Verification items for the finished model (mm, model axes). A direction names the side the tool comes from. Round coordinates to 2 decimals unless told otherwise and drop trailing zeros. Order: outer loops, then holes, each group sorted by start corner. A loop starts at its lowest first (then second) coordinate and runs counter-clockwise, first axis right, second up. Notation, with made-up numbers: M -30.75,61 L 17.25,61 A20 ccw 17.25,67 Z; hole C 42,12.5 d6. An arc over 180 degrees is marked long. Use one line per item in the form item = value. Start each with the question number.
Item 1: Cross-section at A-A on y = 0. Enter the section's corners in (x, z), then the cut area to 3 significant figures.
Item 2: Cross-section at C-C on z = -5.5. Enter the section's corners in (x, y).
Item 3: Tool access check on faces 1 (the flat face through (30.5, 3, -2)), 2 (the flat face through (31.98, -7, -5.33)), 3 (the flat face through (-1.5, 1, -1)), 4 (the flat face through (32, -6.8, -5.1)). Record the directions out of +Z, -Z, +X, -X, +Y, -Y that give a thin tool (end or side, any length) a straight path to the whole face; none if there is none.
Item 4: Cross-section at D-D on x = -12. Enter the section's corners in (y, z).
Item 5: Cross-section at B-B on x = 4. Enter the section's corners in (y, z).
Item 6: Thickness scan on probe 1 along X at (y, z) = (-3.75, -0.5); probe 2 along X at (y, z) = (-1.5, -2.25); probe 3 along Y at (x, z) = (22.5, 5.25). Record the ranges inside material, lowest first. Write a range as [from, to].
Item 7: Go/stop test with flat-tipped pins: pin 1 Ø2 at (x, y) = (-2.5, -6) entering from +Z; pin 2 Ø5.5 at (y, z) = (4, -2) entering from -X; pin 3 Ø10 at (y, z) = (-8.5, 6.5) entering from -X; pin 4 Ø1.8 at (y, z) = (-7, -5) entering from +X. Record where each tip stops, or that it passes through.
from build123d import *

# Parameters (mm, degrees)
EXTRUDE_1_DEPTH = 30.5
SKETCH_2_R      = 3.1
EXTRUDE_2_DEPTH = 1.5
EXTRUDE_START   = -1.5
SKETCH_3_R      = 1
EXTRUDE_3_DEPTH = 23.8
SKETCH_5_R      = 3.15
EXTRUDE_4_DEPTH = 3.2
EXTRUDE_5_DEPTH = 3


with BuildPart() as part:
    # 草图1 → 凸台-拉伸1 (new body)
    with BuildSketch(Plane(origin=(0, 0, 0), x_dir=(0, 0, -1), z_dir=(1, 0, 0))):
        with BuildLine():
            ThreePointArc((-9.15, -7.840918314), (-5.035843242, -10.947272849), (0, -12.05))
            ThreePointArc((0, -12.05), (5.035843242, -10.947272849), (9.15, -7.840918314))
            Line((9.15, -7.840918314), (9.15, 7.840918314))
            ThreePointArc((9.15, 7.840918314), (5.035843234, 10.947272853), (-1.8e-08, 12.05))
            ThreePointArc((-1.8e-08, 12.05), (-5.03584325, 10.947272846), (-9.15, 7.840918314))
            Line((-9.15, 7.840918314), (-9.15, -7.840918314))
        make_face()
    extrude(amount=EXTRUDE_1_DEPTH)

    # 草图2 → 凸台-拉伸2 (add)
    with BuildSketch(Plane.ZY):
        Circle(SKETCH_2_R)
    extrude(amount=EXTRUDE_2_DEPTH)

    # 草图3 → 凸台-拉伸3 (add)
    with BuildSketch(Plane.ZY.offset(1.5).offset(EXTRUDE_START)):
        with Locations(Location((0, 0, 0), (0, 0, 180))):
            Circle(SKETCH_3_R)
    extrude(amount=EXTRUDE_3_DEPTH)

    # 草图5 → 凸台-拉伸4 (add)
    with BuildSketch(Plane(origin=(30.5, 0, 0), x_dir=(0, 0, -1), z_dir=(1, 0, 0))):
        Circle(SKETCH_5_R)
    extrude(amount=EXTRUDE_4_DEPTH)

    # 草图6 → 凸台-拉伸5 (add)
    with BuildSketch(Plane(origin=(30.5, 0, 0), x_dir=(0, 0, -1), z_dir=(1, 0, 0))):
        Polygon((-6.056237864, 6.074082889), (-4.224479128, 7.465003423), (-4.405903545, 7.703928475), (-6.237662281, 6.313007941), align=None)
        Polygon((6.237662281, -6.313007941), (4.405903545, -7.703928475), (4.224479128, -7.465003423), (6.056237864, -6.074082889), align=None)
    extrude(amount=EXTRUDE_5_DEPTH)


solid = part.part
Output values:
q1.outline = M -23.8,-1 L -1.5,-1 L -1.5,-3.1 L 0,-3.1 L 0,-9.15 L 30.5,-9.15 L 30.5,-3.15 L 33.7,-3.15 L 33.7,3.15 L 30.5,3.15 L 30.5,9.15 L 0,9.15 L 0,3.1 L -1.5,3.1 L -1.5,1 L -23.8,1 Z
q1.area = 632 mm2
q2.outline = M 0,-10.72 L 30.5,-10.72 L 30.5,-6.87 L 33.5,-6.87 L 33.5,-6.5 L 30.5,-6.5 L 30.5,10.72 L 0,10.72 Z
q3.face_1 = +X
q3.face_2 = -Z, +X, -Y
q3.face_3 = -X
q3.face_4 = +Z, +X, +Y
q4.outline = C 0,0 d2
q5.outline = M -7.84,-9.15 L 7.84,-9.15 A12.05 ccw 7.84,9.15 L -7.84,9.15 A12.05 ccw Z
q6.probe_1 = [0, 30.5]
q6.probe_2 = [-1.5, 33.7]
q6.probe_3 = [-10.85, 10.85]
q7.pin_1 = through
q7.pin_2 = -1.5
q7.pin_3 = 0
q7.pin_4 = 33.5
